Autodesk Inventor part; units mm, degrees
ref_plane "YZ Plane" through (0, 0, 0) normal (1, 0, 0) x (0, 1, 0)
ref_plane "XZ Plane" through (0, 0, 0) normal (0, 1, 0) x (-1, 0, 0)
ref_plane "XY Plane" through (0, 0, 0) normal (0, 0, 1) x (1, 0, 0)
sketch "Sketch1" plane through (0, 0, 0) normal (1, 0, 0) x (0, 1, 0)
  line L0 (23.4698, 23.9871) -> (-20.5302, 23.9871)
  line L1 (-20.5302, 23.9871) -> (-20.5302, -41.0129)
  line L2 (-20.5302, -41.0129) -> (23.4698, -41.0129)
  line L3 (23.4698, -41.0129) -> (23.4698, 23.9871)
  point P0 (0, 0)
  dimension "d0" = 44
  dimension "d1" = 65
extrude "Extrusion1" add sketch "Sketch1" along normal blind 12
sketch "Sketch2" plane through (12, 0, 0) normal (1, 0, 0) x (0, 0, -1)
  line L0 (-13.9871, 13.4698) -> (31.0129, 13.4698)
  line L1 (31.0129, 13.4698) -> (31.0129, -10.5602)
  line L2 (31.0129, -10.5602) -> (-13.9871, -10.5602)
  line L3 (-13.9871, -10.5602) -> (-13.9871, 13.4698)
  line L4 (41.0129, 23.4698) -> (-23.9871, 23.4698)
  line L5 (-23.9871, 23.4698) -> (-23.9871, -20.5302)
  point P0 (0, 0)
  dimension "d4" = 24.03
  dimension "d5" = 10
  dimension "d6" = 10
  dimension "d7" = 45
extrude "Extrusion2" cut sketch "Sketch2" against normal blind 50.1
sketch "Sketch3" plane through (12, 0, 0) normal (1, 0, 0) x (0, 0, -1)
  line L0 (-23.9871, -20.5302) -> (41.0129, -20.5302)
  line L1 (41.0129, 23.4698) -> (-23.9871, 23.4698)
  line L2 (41.0129, -20.5302) -> (41.0129, 23.4698)
  point P0 (0, 0)
  point P1 (11.0129, 18.4698)
  point P2 (11.0129, -15.5302)
  dimension "d10" = 0
  dimension "d11" = 5
  dimension "d12" = 5
  dimension "d13" = 30
hole "Hole1" at (12, 18.4698, -11.0129) at (12, -15.5302, -11.0129) direction (-1, 0, 0) diameter 2.4638 end through all
sketch "Sketch4" plane through (0, 23.4698, 23.9871) normal (0, 1, 0) x (1, 0, 0)
  line L0 (0, 0) -> (12, 0)
  line L1 (0, 65) -> (12, 65)
  line L2 (0, 65) -> (0, 0)
  point P0 (0, 23.9871)
  point P1 (6, 5)
  point P2 (6, 60)
  dimension "d21" = 0
  dimension "d22" = 5
  dimension "d23" = 5
  dimension "d24" = 6
hole "Hole2" at (6, 23.4698, 18.9871) at (6, 23.4698, -36.0129) direction (0, -1, 0) diameter 2.4638 end through all
sketch "Sketch5" plane through (0, -20.5302, 23.9871) normal (0, 0, 1) x (1, 0, 0)
  line L0 (0, 44) -> (12, 44)
  line L1 (0, 0) -> (12, 0)
  line L2 (0, 44) -> (0, 0)
  point P0 (0, 20.5302)
  point P1 (6, 5)
  point P2 (6, 39)
  dimension "d32" = 0
  dimension "d33" = 5
  dimension "d34" = 5
  dimension "d35" = 6
hole "Hole3" at (6, -15.5302, 23.9871) at (6, 18.4698, 23.9871) direction (0, 0, -1) diameter 2.4638 end through all
properties part number "LidarV4Mount"
The listing builds one solid part. Answer for the finished solid, in the listing's coordinates (mm). A direction names the side the tool comes from. Coordinates: 2 decimals unless noted, no trailing zeros. Write each loop counter-clockwise with the first axis right and the second up, starting at its lowest first coordinate (ties: lowest second). Pieces come first, ordered by that corner, then holes. Notation, with made-up numbers: M 73.5,-39.5 L 86.5,-39.5 A11 ccw 86.5,-29.5 Z; hole C 1.5,60.25 d3. An arc over 180 degrees is marked long. Put each result on its own line as item: value. Start each with the question number.
1. Consider line 1 (Y direction, x = 6, z = -38.8); line 2 (Z direction, x = 3, y = -6); line 3 (Y direction, x = 11.5, z = -22). Determine where each line is inside the solid, lowest interval first. Write a range as from..to.
2. Which of the six approach directions +Z, -Z, +X, -X, +Y, -Y give full straight-line access (tool end or side, diameter ignored) to faces 1 (the flat face through (6, -10.56, -9)), 2 (the cylindrical face through (5.63, 17.295, -39.103))?
3. For a pull along Z with two mould halves and no side action, classify faces 3 (the cylindrical face through (4.96, 17.81, 22.01)), 4 (the flat face through (6, 1, 13.987)), 5 (the flat face through (6, 1, -41.013)), 6 (the cylindrical face through (5.946, 1.232, -37.244)) as pulls with the +Z half, pulls with the -Z half, needs draft (parallel to the pull), parting line crosses it, or undercut.
4. A cutting plane is placed at A-A on y = -1. Write down the section's boundary in (x, z), then the cut area to 3 significant figures.
5. A cutting plane is placed at B-B on z = -23. Write down the section's boundary in (x, y), then the cut area to 3 significant figures.
6. A cutting plane is placed at C-C on x = 10.5. Write down the section's boundary in (y, z).
Resolved:
1. line 1: y = -20.53..-16.76, -14.3..17.24, 19.7..23.47
1. line 2: z = -41.01..-31.01, 13.99..23.99
1. line 3: y = -20.53..-10.56, 13.47..23.47
2. face 1: +X, -X
2. face 2: +Z, -Z
3. face 3: needs draft
3. face 4: undercut
3. face 5: pulls with the -Z half
3. face 6: undercut
4. outline: M 0,-41.01 L 12,-41.01 L 12,-31.01 L 0,-31.01 Z; M 0,13.99 L 12,13.99 L 12,23.99 L 0,23.99 Z; hole C 6,-36.01 d2.46; hole C 6,18.99 d2.46
4. area: 230 mm2
5. outline: M 0,-20.53 L 12,-20.53 L 12,-10.56 L 0,-10.56 Z; M 0,13.47 L 12,13.47 L 12,23.47 L 0,23.47 Z; hole C 6,-15.53 d2.46; hole C 6,18.47 d2.46
5. area: 230 mm2
6. outline: M -20.53,-41.01 L 23.47,-41.01 L 23.47,23.99 L -20.53,23.99 Z; hole C -15.53,-11.01 d2.46; hole M -10.56,-31.01 L 13.47,-31.01 L 13.47,13.99 L -10.56,13.99 Z; hole C 18.47,-11.01 d2.46
